The model under review builds one solid part; all positions refer to its coordinate system, in mm. Face numbers are marked on the shaded views. Round coordinates to 2 decimals unless told otherwise and drop trailing zeros. Loops run counter-clockwise (first coordinate to the right, second up) from the corner with the lowest first, then second, coordinate; pieces in that order, holes last. Notation, with made-up numbers: M 22.25,-40 L 38.25,-40 A14 ccw 38.25,-35 Z; hole C 21.5,6.25 d8. An arc over 180 degrees is marked long. Use a Markdown table: item, result. Add a question column.
```python
from build123d import *

# Parameters (mm, degrees)
SKETCH1_R           = 80
BOSS_EXTRUDE1_DEPTH = 2
CUT_EXTRUDE1_DEPTH  = 2
SKETCH3_R           = 2.5
CUT_EXTRUDE2_DEPTH  = 114.154761279
SKETCH4_W           = 105
SKETCH4_H           = 22
SKETCH4_W_2         = 95
SKETCH4_H_2         = 12
BOSS_EXTRUDE2_DEPTH = 3
CUT_EXTRUDE3_DEPTH  = 146.976025429
FILLET1_R           = 10
SKETCH6_R           = 2
CUT_EXTRUDE4_DEPTH  = 114.176852757
MOVE_FACE1_BY       = 0.2
MOVE_FACE1_2_BY     = 0.2
MOVE_FACE1_3_BY     = 0.2
MOVE_FACE1_4_BY     = 0.2
SKETCH7_R           = 10.6
CUT_EXTRUDE5_DEPTH  = 114.176852757


with BuildPart() as part:
    # Sketch1 → Boss-Extrude1 (new body)
    with BuildSketch(Plane(origin=(0, 0, 0), x_dir=(1, 0, 0), z_dir=(0, 1, 0))):
        with Locations(Location((0, 0, 0), (0, 0, 270))):
            Circle(SKETCH1_R)
    extrude(amount=BOSS_EXTRUDE1_DEPTH)

    # Sketch2 → Cut-Extrude1 (cut)
    with BuildSketch(Plane(origin=(0, 2, 0), x_dir=(1, 0, 0), z_dir=(0, 1, 0))):
        with BuildLine():
            ThreePointArc((-66.565172984, -11.19498752), (-69.445178929, -9.14423991), (-71.495926539, -12.024245855))
            ThreePointArc((-71.495926539, -12.024245855), (-51.265241636, -51.265241636), (-12.024245855, -71.495926539))
            ThreePointArc((-12.024245855, -71.495926539), (-9.14423991, -69.445178929), (-11.19498752, -66.565172984))
            ThreePointArc((-11.19498752, -66.565172984), (-47.72970773, -47.72970773), (-66.565172984, -11.19498752))
        make_face()
        with BuildLine():
            ThreePointArc((-66.565172984, 11.19498752), (-69.445178929, 9.14423991), (-71.495926539, 12.024245855))
            ThreePointArc((-71.495926539, 12.024245855), (-51.265241636, 51.265241636), (-12.024245855, 71.495926539))
            ThreePointArc((-12.024245855, 71.495926539), (-9.14423991, 69.445178929), (-11.19498752, 66.565172984))
            ThreePointArc((-11.19498752, 66.565172984), (-47.72970773, 47.72970773), (-66.565172984, 11.19498752))
        make_face()
        with BuildLine():
            ThreePointArc((11.19498752, -66.565172984), (9.14423991, -69.445178929), (12.024245855, -71.495926539))
            ThreePointArc((12.024245855, -71.495926539), (51.265241636, -51.265241636), (71.495926539, -12.024245855))
            ThreePointArc((71.495926539, -12.024245855), (69.445178929, -9.14423991), (66.565172984, -11.19498752))
            ThreePointArc((66.565172984, -11.19498752), (47.72970773, -47.72970773), (11.19498752, -66.565172984))
        make_face()
        with BuildLine():
            ThreePointArc((66.565172984, 11.19498752), (69.445178929, 9.14423991), (71.495926539, 12.024245855))
            ThreePointArc((71.495926539, 12.024245855), (51.265241636, 51.265241636), (12.024245855, 71.495926539))
            ThreePointArc((12.024245855, 71.495926539), (9.14423991, 69.445178929), (11.19498752, 66.565172984))
            ThreePointArc((11.19498752, 66.565172984), (47.72970773, 47.72970773), (66.565172984, 11.19498752))
        make_face()
    extrude(amount=-CUT_EXTRUDE1_DEPTH, mode=Mode.SUBTRACT)

    # Sketch3 → Cut-Extrude2 (cut, through all)
    with BuildSketch(Plane(origin=(0, 2, 0), x_dir=(1, 0, 0), z_dir=(0, 1, 0))):
        with Locations(Location((-44.5, -31, 0), (0, 0, 270))):
            Circle(SKETCH3_R)
        with Locations(Location((44.5, -31, 0), (0, 0, 270))):
            Circle(SKETCH3_R)
    extrude(amount=-CUT_EXTRUDE2_DEPTH, mode=Mode.SUBTRACT)

    # Sketch4 → Boss-Extrude2 (add)
    with BuildSketch(Plane(origin=(0, 2, 0), x_dir=(1, 0, 0), z_dir=(0, 1, 0))):
        with Locations((0, -31)):
            Rectangle(SKETCH4_W, SKETCH4_H)
        with Locations((0, -31)):
            Rectangle(SKETCH4_W_2, SKETCH4_H_2, mode=Mode.SUBTRACT)
    extrude(amount=BOSS_EXTRUDE2_DEPTH)

    # Sketch5 → Cut-Extrude3 (cut, through all)
    with BuildSketch(Plane.XY.offset(42)):
        Polygon((0, 2), (-10, 5), (10, 5), align=None)
    extrude(amount=-CUT_EXTRUDE3_DEPTH, mode=Mode.SUBTRACT)

    # Fillet1
    # the kernel refuses this fillet: 10 mm, written as the material it adds along each edge
    with BuildSketch(Plane(origin=(0, 2, 25), x_dir=(-0.9578262852211515, 0.2873478855663449, 0), z_dir=(0, 0, -1)), Plane(origin=(0, 2, 42), x_dir=(-0.9578262852211515, 0.2873478855663449, 0), z_dir=(0, 0, -1))) as fillet1_piece_1:
        with BuildLine():
            CenterArc((FILLET1_R * 0.3, FILLET1_R), FILLET1_R, 236.601511532, 33.398488468)
            Line((-FILLET1_R * 0.250458715596, FILLET1_R * 0.165137614679), (0, 0))
            Line((0, 0), (FILLET1_R * 0.3, 0))
        make_face()
    extrude(amount=5)
    # the kernel refuses this fillet: 10 mm, written as the material it takes off along each edge
    with BuildSketch(Plane(origin=(10, 5, 28.669220908), x_dir=(-0.9578262852211505, -0.28734788556634844, 0), z_dir=(0, 0, -1)), Plane(origin=(-10, 5, 28.669220908), x_dir=(-1, 0, 0), z_dir=(0, 0, -1)), Plane(origin=(-10, 5, 45.669220908), x_dir=(-1, 0, 0), z_dir=(0, 0, -1))) as fillet1_2_piece_1:
        with BuildLine():
            CenterArc((FILLET1_R * 0.146768836304, -FILLET1_R), FILLET1_R, 90, 16.699244234)
            Line((-FILLET1_R * 0.140579049263, -FILLET1_R * 0.0421737147788), (0, 0))
            Line((0, 0), (FILLET1_R * 0.146768836304, 0))
        make_face()
    extrude(amount=12.338441815, mode=Mode.SUBTRACT)
    with BuildSketch(Plane(origin=(10, 5, 45.669220908), x_dir=(1, 0, 0), z_dir=(0, 0, -1))) as fillet1_2_piece_2:
        with BuildLine():
            CenterArc((FILLET1_R * 0.146768836304, FILLET1_R), FILLET1_R, 253.300755766, 16.699244234)
            Line((-FILLET1_R * 0.140579049263, FILLET1_R * 0.0421737147788), (0, 0))
            Line((0, 0), (FILLET1_R * 0.146768836304, 0))
        make_face()
    extrude(amount=12.338441815, mode=Mode.SUBTRACT)

    # Sketch6 → Cut-Extrude4 (cut, through all)
    with BuildSketch(Plane(origin=(0, 2, 0), x_dir=(1, 0, 0), z_dir=(0, 1, 0))):
        with Locations(Location((42.5, 63, 0), (0, 0, 270))):
            Circle(SKETCH6_R)
        with Locations(Location((42.5, 21, 0), (0, 0, 270))):
            Circle(SKETCH6_R)
        with Locations(Location((-42.5, 21, 0), (0, 0, 90))):
            Circle(SKETCH6_R)
        with Locations(Location((-42.5, 63, 0), (0, 0, 90))):
            Circle(SKETCH6_R)
    extrude(amount=-CUT_EXTRUDE4_DEPTH, mode=Mode.SUBTRACT)

    # Move Face1: a face moved inward by 0.2
    extrude(part.faces().sort_by_distance((47.5, 3.5, 31))[0], amount=MOVE_FACE1_BY, dir=(1, 0, 0), mode=Mode.SUBTRACT)

    # Move Face1 2: a face moved inward by 0.2
    extrude(part.faces().sort_by_distance((0, 2.3, 37))[0], amount=MOVE_FACE1_2_BY, dir=(0, 0, 1), mode=Mode.SUBTRACT)

    # Move Face1 3: a face moved inward by 0.2
    extrude(part.faces().sort_by_distance((-47.5, 3.5, 31))[0], amount=MOVE_FACE1_3_BY, dir=(-1, 0, 0), mode=Mode.SUBTRACT)

    # Move Face1 4: a face moved inward by 0.2
    extrude(part.faces().sort_by_distance((-24.162844037, 2.873853211, 25))[0], amount=MOVE_FACE1_4_BY, dir=(0, 0, -1), mode=Mode.SUBTRACT)

    # Sketch7 → Cut-Extrude5 (cut, through all)
    with BuildSketch(Plane(origin=(0, 2, 0), x_dir=(1, 0, 0), z_dir=(0, 1, 0))):
        with Locations(Location((0, 0, 0), (0, 0, 270))):
            Circle(SKETCH7_R)
    extrude(amount=-CUT_EXTRUDE5_DEPTH, mode=Mode.SUBTRACT)


solid = part.part
```
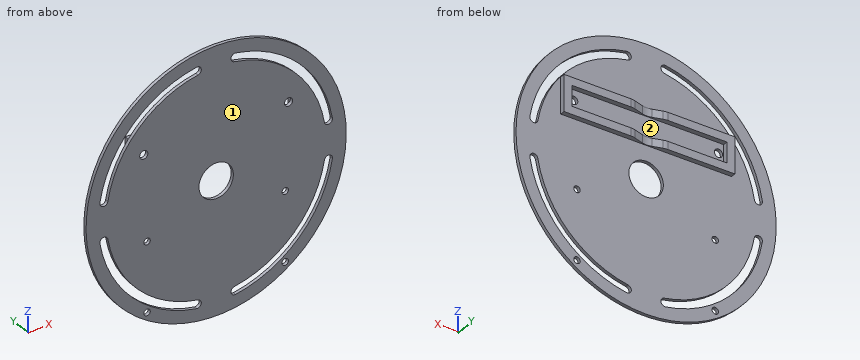
(1) Consider section C-C, the plane z = -47.5. Give the boundary of the cut face in (x, y).
(2) Consider section D-D, the plane x = 0. Give the boundary of the cut face in (y, z).
(3) Consider section B-B, the plane x = -62. Give the boundary of the cut face in (y, z).
(4) Insertion check: pin 1 Ø4.5 at (x, z) = (42.5, -21) entering from +Y; pin 2 Ø2 at (x, z) = (17.5, -24) entering from -Y; pin 3 Ø2 at (x, y) = (-4.5, 2.5) entering from +Z; pin 4 Ø13.5 at (x, z) = (-5, 33.5) entering from +Y. Each pin has a flat end and moves straight along its axis. Give the tip position at first contact, or say it passes through.
(5) To check wall thickness, follow probe 1 along Z at (x, y) = (-38, 4.75); probe 2 along Z at (x, y) = (-41, 1.95); probe 3 along X at (y, z) = (1.4, 51.5). State the ranges of each line that lie inside material, in increasing order.
(6) Draft analysis for pull direction Z (two halves, no side actions). For the marked faces 1 and 2, state which applies: released by +Z, released by -Z, zero draft, split by the parting line, or undercut.
(7) Consider section A-A, the plane y = 1.2. Give the number of separate pieces and of enclosed holes in the cut face, then the cut area to 3 significant figures.
Found:
| question | item | result |
|---|---|---|
| 1 | outline | M -64.37,0 L -54.77,0 L -54.77,2 L -64.37,2 Z; M -47.96,0 L 47.96,0 L 47.96,2 L -47.96,2 Z; M 54.77,0 L 64.37,0 L 64.37,2 L 54.77,2 Z |
| 2 | outline | M 0,-80 L 2,-80 L 2,-10.6 L 0,-10.6 Z; M 0,10.6 L 2,10.6 L 2,20 L 2.44,20 L 2.44,24.8 L 2,24.8 L 2,37.2 L 2.44,37.2 L 2.44,42 L 2,42 L 2,80 L 0,80 Z |
| 3 | outline | M 0,-50.56 L 2,-50.56 L 2,-37.58 L 0,-37.58 Z; M 0,-26.69 L 2,-26.69 L 2,26.69 L 0,26.69 Z; M 0,37.58 L 2,37.58 L 2,50.56 L 0,50.56 Z |
| 4 | pin 1 | stops at y = 2 |
| 4 | pin 2 | stops at y = 0 |
| 4 | pin 3 | stops at z = 79.92 |
| 4 | pin 4 | stops at y = 4.97 |
| 5 | probe 1 | z = 20 to 24.8, 37.2 to 42 |
| 5 | probe 2 | z = -68.69 to -64.32, -61.68 to -59.79, -53.62 to -22.32, -19.68 to 53.62, 59.79 to 68.69 |
| 5 | probe 3 | x = -61.22 to -51.03, -43.63 to 43.63, 51.03 to 61.22 |
| 6 | face 1 | zero draft |
| 6 | face 2 | undercut |
| 7 | separate pieces | 1 |
| 7 | enclosed holes | 11 |
| 7 | area | 17,900 mm^2 |
